from build123d import *

# Parameters (mm, degrees)
SKETCH_1_W                = 10
SKETCH_1_H                = 30
EXTRUDE_1_DEPTH           = 10
HOLE_WIZARD_1_D           = 4.5
HOLE_WIZARD_1_CBORE_D     = 8
HOLE_WIZARD_1_CBORE_DEPTH = 4.6
HOLE_WIZARD_M5_1_D        = 4.2
SKETCH_6_R                = 4.5
CUT_EXTRUDE_1_DEPTH       = 5


with BuildPart() as part:
    # 草图1 → 凸台-拉伸1 (new body)
    with BuildSketch(Plane.XY):
        Rectangle(SKETCH_1_W, SKETCH_1_H)
    extrude(amount=EXTRUDE_1_DEPTH)

    # 打孔尺寸(%根据)内六角圆柱头螺钉的类型1 (through all)
    with Locations(Plane.XY.offset(10)):
        with Locations((0, 10), (0, -10)):
            CounterBoreHole(HOLE_WIZARD_1_D / 2, HOLE_WIZARD_1_CBORE_D / 2, HOLE_WIZARD_1_CBORE_DEPTH)

    # M5 螺纹孔1 (through all)
    with Locations(Plane(origin=(5, 0, 0), x_dir=(0, 0, -1), z_dir=(1, 0, 0))):
        with Locations((-5, 0)):
            Hole(HOLE_WIZARD_M5_1_D / 2)

    # 草图6 → 切除-拉伸1 (cut)
    with BuildSketch(Plane(origin=(5, 0, 0), x_dir=(0, 0, -1), z_dir=(1, 0, 0))):
        with Locations((-5, 0)):
            Circle(SKETCH_6_R)
    extrude(amount=-CUT_EXTRUDE_1_DEPTH, mode=Mode.SUBTRACT)


solid = part.part
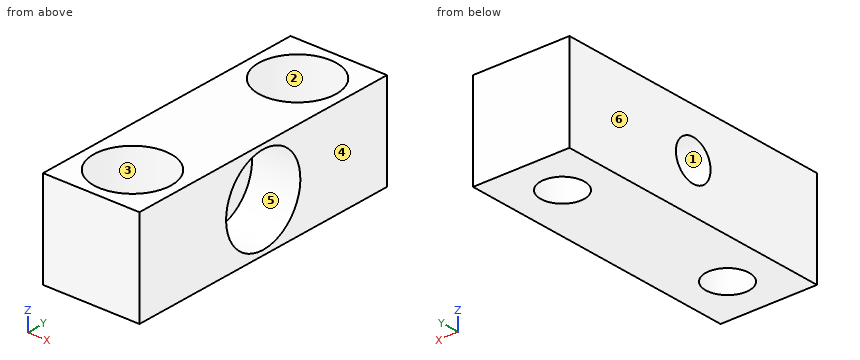
Can you work these out from the model? Positions are in its coordinate system, mm. Face numbers are marked on the shaded views. A direction names the side the tool comes from. Give positions to 0.01 mm unless a question says otherwise; leave off trailing zeros. Order: outer loops, then holes, each group sorted by start corner. A loop starts at its lowest first (then second) coordinate and runs counter-clockwise, first axis right, second up. Notation, with made-up numbers: M 57.25,65 L 110.25,65 A26 ccw 110.25,91 Z; hole C 3.5,-25 d1. An arc over 180 degrees is marked long. Use one line per item in the form item = value. Start each with the question number.
Item 1: If we section it at A-A (z = 5): Write out the boundary of the cut face in (x, y), then the cut area to 3 significant figures.
Item 2: For the marked faces 1 and 2, which set-ups out of +Z, -Z, +X, -X, +Y, -Y let a thin tool reach every point of the face, with its end or its side?
Item 3: If we section it at B-B (y = 0): Write out the boundary of the cut face in (x, z), then the cut area to 3 significant figures.
Item 4: Will these pins go through, and if not, where does the flat tip stop? pin 1 Ø4.5 at (y, z) = (0.5, 3.5) entering from +X; pin 2 Ø2.5 at (x, y) = (2, 8) entering from +Z; pin 3 Ø4 at (x, y) = (0.5, -11.5) entering from +Z.
Item 5: If I drill on line 1 along Y through (x, z) = (-0.5, 7.5); line 2 along Y through (x, z) = (0.5, 4.5); line 3 along Y through (x, z) = (0.5, 4), over which ranges is the centre line in solid material (lowest first)?
Item 6: We'd pull the mould along X, two halves only. Please class the marked faces 3, 4, 5 and 6: +X half, -X half, draft (parallel to the pull), parting line (faces both ways), or undercut.
Item 7: If we section it at C-C (x = -1): Write out the boundary of the cut face in (y, z).
Item 8: If we section it at D-D (z = 1.75): Write out the boundary of the cut face in (x, y).
Outcome:
q1.outline = M -5,-15 L 5,-15 L 5,-4.5 L 0,-4.5 L 0,-2.1 L -5,-2.1 Z; M -5,2.1 L 0,2.1 L 0,4.5 L 5,4.5 L 5,15 L -5,15 Z; hole C 0,-10 d4.5; hole C 0,10 d4.5
q1.area = 202 mm2
q2.face_1 = +X, -X
q2.face_2 = +Z
q3.outline = M -5,0 L 5,0 L 5,0.5 L 0,0.5 L 0,2.9 L -5,2.9 Z; M -5,7.1 L 0,7.1 L 0,9.5 L 5,9.5 L 5,10 L -5,10 Z
q3.area = 34.0 mm2
q4.pin_1 = 0
q4.pin_2 = 10
q4.pin_3 = 5.4
q5.line_1 = -15 to -13.97, -6.03 to 6.03, 13.97 to 15
q5.line_2 = -15 to -12.19, -7.81 to -4.47, 4.47 to 7.81, 12.19 to 15
q5.line_3 = -15 to -12.19, -7.81 to -4.39, 4.39 to 7.81, 12.19 to 15
q6.face_3 = undercut
q6.face_4 = +X half
q6.face_5 = draft
q6.face_6 = -X half
q7.outline = M -15,0 L -12.02,0 L -12.02,5.4 L -13.87,5.4 L -13.87,10 L -15,10 Z; M -7.98,0 L 7.98,0 L 7.98,5.4 L 6.13,5.4 L 6.13,10 L -6.13,10 L -6.13,5.4 L -7.98,5.4 Z; M 12.02,0 L 15,0 L 15,10 L 13.87,10 L 13.87,5.4 L 12.02,5.4 Z; hole C 0,5 d4.2
q8.outline = M -5,-15 L 5,-15 L 5,-3.11 L 0,-3.11 L 0,3.11 L 5,3.11 L 5,15 L -5,15 Z; hole C 0,-10 d4.5; hole C 0,10 d4.5
